```python
from build123d import *

# Parameters (mm, degrees)
SKETCH9_R           = 6.65
BOSS_EXTRUDE1_DEPTH = 39.9


with BuildPart() as part:
    # Sketch9 → Boss-Extrude1 (new body)
    with BuildSketch(Plane(origin=(0, 0, 0), x_dir=(0, 1, 0), z_dir=(0, 0, 1))):
        with BuildLine():
            Line((800, 286.45), (411.016496764, 7.889188745))
            ThreePointArc((411.016496764, 7.889188745), (407.294864157, -11.41873272), (388.21106152, -6.680077058))
            Line((388.21106152, -6.680077058), (11.78893848, -6.680077058))
            ThreePointArc((11.78893848, -6.680077058), (2.770053686, -13.263834384), (-8.13, -10.84))
            Line((-8.13, -10.84), (-408.13, 289.16))
            ThreePointArc((-408.13, 289.16), (-410.355747525, 308.738477739), (-390.681827116, 309.837385532))
            Line((-390.681827116, 309.837385532), (790.681827116, 309.837385532))
            ThreePointArc((790.681827116, 309.837385532), (812.58767401, 305.015272976), (800, 286.45))
        make_face()
        with Locations(Location((-400, 300, 0), (0, 0, 270))):
            Circle(SKETCH9_R, mode=Mode.SUBTRACT)
        with Locations(Location((0, 0, 0), (0, 0, 270))):
            Circle(SKETCH9_R, mode=Mode.SUBTRACT)
        with Locations(Location((400, 0, 0), (0, 0, 270))):
            Circle(SKETCH9_R, mode=Mode.SUBTRACT)
        with Locations(Location((800, 300, 0), (0, 0, 270))):
            Circle(SKETCH9_R, mode=Mode.SUBTRACT)
        with BuildLine():
            Line((-386.45, 300), (393.040410471, 11.626117735))
            ThreePointArc((393.040410471, 11.626117735), (396.389694979, 13.060176019), (400, 13.55))
            Line((400, 13.55), (786.45, 300))
            Line((786.45, 300), (-386.45, 300))
        make_face(mode=Mode.SUBTRACT)
        with BuildLine():
            Line((-390.681827116, 290.162614468), (368.558996023, 6.680077058))
            Line((368.558996023, 6.680077058), (11.78893848, 6.680077058))
            ThreePointArc((11.78893848, 6.680077058), (2.770053686, 13.263834384), (-8.13, 10.84))
            Line((-8.13, 10.84), (-390.681827116, 290.162614468))
        make_face(mode=Mode.SUBTRACT)
    extrude(amount=BOSS_EXTRUDE1_DEPTH)


solid = part.part
```
Read the model definition and answer for the solid it produces. Units are mm, in the model's axes. A direction names the side the tool comes from. Give positions to 0.01 mm unless a question says otherwise; leave off trailing zeros. Order: outer loops, then holes, each group sorted by start corner. A loop starts at its lowest first (then second) coordinate and runs counter-clockwise, first axis right, second up.
(1) Find section D-D (y = -59). Give the vertices of the cut face in (x, z).
(2) Straight lines are drawn through the part: L1, parallel to X at y = 252, z = 6.5; L2, parallel to X at y = 800, z = 12; L3, parallel to X at y = 188, z = 33. For each, find the intervals that lie inside material, in ascending order.
(3) For faces 5 (the flat face through (-114, 112, 0)), 6 (the flat face through (-309.837, 192, 20)), 7 (the flat face through (6.68, 203, 20)), 8 (the flat face through (-157.83, -2.16, 19.67)), determine the directions among +Z, -Z, +X, -X, +Y, -Y from which every point of the face is accessible in a straight line to the end or side of a thin tool.
(4) Find section B-B (x = -244). Give the vertices of the cut face in (y, z), plus the area to 3 significant figures.
(5) Find section A-A (z = 24). Give the vertices of the cut face in (x, y).
(6) For a pull along Y with two mould halves and no side action, classify faces 1 (the flat face through (-137.06, -205.33, 19.67)), 2 (the flat face through (-149.12, 608.23, 19.67)), 3 (the flat face through (-148.546, -196.728, 19.671)), 4 (the flat face through (-114, 112, 39.9)) as released by +Y, released by -Y, zero draft, split by the parting line, or undercut.
(7) Given pin 1 (5 mm diameter, centred on y = -74, z = 12, fed in from -X); pin 2 (12 mm diameter, centred on y = 226.5, z = 30, fed in from +X); pin 3 (17.5 mm diameter, centred on x = 0, y = 400, fed in from +Z); pin 4 (6 mm diameter, centred on x = -45.5, z = 30.5, fed in from +Y), each flat-ended and moving along its own axis, determine where each tip first touches the part or whether it passes through.
(8) Find section C-C (y = 709.5). Give the vertices of the cut face in (x, z), plus the area to 3 significant figures.
Result sheet:
1. outline: (-309.84, 0) - (-300, 0) - (-300, 39.9) - (-309.84, 39.9) - close; (-178.86, 0) - (-166.32, 0) - (-166.32, 39.9) - (-178.86, 39.9) - close; (-47.98, 0) - (-27.31, 0) - (-27.31, 39.9) - (-47.98, 39.9) - close
2. L1: x = -309.84 to -300, -63.8 to -50.2, -6.68 to 6.68
2. L2: x = -313.55 to -306.65, -293.35 to -286.45
2. L3: x = -309.84 to -300, -87.48 to -74.1, -6.68 to 6.68
3. face 5: -Z, +X, -X, +Y, -Y
3. face 6: +Z, -Z, -X
3. face 7: +Z, -Z, +X
3. face 8: +Z, -Z
4. outline: (-347.92, 0) - (-327.46, 0) - (-327.46, 39.9) - (-347.92, 39.9) - close; (-267.05, 0) - (-235.08, 0) - (-235.08, 39.9) - (-267.05, 39.9) - close; (710.9, 0) - (740.72, 0) - (740.72, 39.9) - (710.9, 39.9) - close
4. area: 3,280 mm2
5. outline: (-309.84, -390.68) arc R13.55 ccw (long way) to (-289.16, -408.13) - (10.84, -8.13) arc R13.55 ccw to (6.68, 11.79) - (6.68, 388.21) arc R13.55 ccw (long way) to (-7.89, 411.02) - (-286.45, 800) arc R13.55 ccw (long way) to (-309.84, 790.68) - close; hole circle Ø13.3 at (-300, -400); hole circle Ø13.3 at (-300, 800); hole (-300, -386.45) - (-11.63, 393.04) arc R13.55 cw to (-13.55, 400) - (-300, 786.45) - close; hole (-290.16, -390.68) - (-10.84, -8.13) arc R13.55 cw to (-6.68, 11.79) - (-6.68, 368.56) - close; hole circle Ø13.3 at (0, 0); hole circle Ø13.3 at (0, 400)
6. face 1: released by -Y
6. face 2: released by +Y
6. face 3: undercut
6. face 4: zero draft
7. pin 1: stops at x = -309.84
7. pin 2: stops at x = 6.68
7. pin 3: stops at z = 39.9
7. pin 4: stops at y = 467.73
8. outline: (-309.84, 0) - (-300, 0) - (-300, 39.9) - (-309.84, 39.9) - close; (-242.96, 0) - (-221.64, 0) - (-221.64, 39.9) - (-242.96, 39.9) - close
8. area: 1,240 mm2
